from build123d import *

# Parameters (mm, degrees)
EXTRUDE_1_DEPTH     = 15
EXTRUDE_1_2_DEPTH   = 15
EXTRUDE_2_DEPTH     = 4
EXTRUDE_5_DEPTH     = 4
SKETCH_8_W          = 5
SKETCH_8_H          = 5
EXTRUDE_6_DEPTH     = 37
SKETCH_9_W          = 4
SKETCH_9_H          = 5
EXTRUDE_7_DEPTH     = 60
EXTRUDE_8_DEPTH     = 5
FILLET_1_R          = 1
FILLET_2_R          = 1
SKETCH_11_W         = 94.407997399
SKETCH_11_H         = 0.2
CUT_EXTRUDE_1_DEPTH = 61


with BuildPart() as part:
    # Sketch 1 → Extrude 1 (new body)
    with BuildSketch(Plane.XY):
        with BuildLine():
            Line((539.301234579, 452.744075086), (539.301234579, 447.744075086))
            Line((539.301234579, 447.744075086), (534.301234579, 447.744075086))
            ThreePointArc((534.301234579, 447.744075086), (531.801234579, 450.244075086), (534.301234579, 452.744075086))
            Line((534.301234579, 452.744075086), (539.301234579, 452.744075086))
        make_face()
    extrude(amount=-EXTRUDE_1_DEPTH)



with BuildPart() as body_2:
    # Sketch 1 → Extrude 1 2 (new body)
    with BuildSketch(Plane.XY):
        with BuildLine():
            Line((459.301234579, 452.744075086), (459.301234579, 447.744075086))
            Line((459.301234579, 447.744075086), (454.301234579, 447.744075086))
            ThreePointArc((454.301234579, 447.744075086), (451.801234579, 450.244075086), (454.301234579, 452.744075086))
            Line((454.301234579, 452.744075086), (459.301234579, 452.744075086))
        make_face()
    extrude(amount=-EXTRUDE_1_2_DEPTH)


with BuildPart() as part_1:
    add(part.part)

    add(body_2.part)  # Extrude 2 merges body 2
    # Sketch 2 → Extrude 2 (add)
    with BuildSketch(Plane(origin=(0, 0, -15), x_dir=(-1, 0, 0), z_dir=(0, 0, -1))):
        with BuildLine():
            Line((-529.301234579, 452.744075086), (-534.301234579, 452.744075086))
            Line((-534.301234579, 452.744075086), (-539.301234579, 452.744075086))
            Line((-539.301234579, 452.744075086), (-539.301234579, 447.744075086))
            Line((-539.301234579, 447.744075086), (-534.301234579, 447.744075086))
            Line((-534.301234579, 447.744075086), (-529.301234579, 447.744075086))
            ThreePointArc((-529.301234579, 447.744075086), (-526.801234579, 450.244075086), (-529.301234579, 452.744075086))
        make_face()
        with BuildLine():
            Line((-449.301234579, 452.744075086), (-459.301234579, 452.744075086))
            Line((-459.301234579, 452.744075086), (-459.301234579, 447.744075086))
            Line((-459.301234579, 447.744075086), (-449.301234579, 447.744075086))
            ThreePointArc((-449.301234579, 447.744075086), (-446.801234579, 450.244075086), (-449.301234579, 452.744075086))
        make_face()
    extrude(amount=EXTRUDE_2_DEPTH)

    # Sketch 7 → Extrude 5 (add)
    with BuildSketch(Plane.XY):
        with BuildLine():
            Line((539.301234579, 447.744075086), (454.301234579, 447.744075086))
            ThreePointArc((454.301234579, 447.744075086), (451.801234579, 450.244075086), (454.301234579, 452.744075086))
            Line((454.301234579, 452.744075086), (539.301234579, 452.744075086))
            Line((539.301234579, 452.744075086), (539.301234579, 447.744075086))
        make_face()
    extrude(amount=EXTRUDE_5_DEPTH)

    # Sketch 8 → Extrude 6 (add)
    with BuildSketch(Plane.XY.offset(4)):
        with Locations((536.801234579, 450.244075086)):
            Rectangle(SKETCH_8_W, SKETCH_8_H)
        with Locations((476.801234579, 450.244075086)):
            Rectangle(SKETCH_8_W, SKETCH_8_H)
    extrude(amount=EXTRUDE_6_DEPTH)

    # Sketch 9 → Extrude 7 (add)
    with BuildSketch(Plane.ZY.offset(-534.301234579)):
        with Locations((39, 450.244075086)):
            Rectangle(SKETCH_9_W, SKETCH_9_H)
    extrude(amount=EXTRUDE_7_DEPTH)

    # Sketch 10 → Extrude 8 (add)
    with BuildSketch(Plane.XZ.offset(-447.744075086)):
        Polygon((474.301234579, 4), (469.301234579, 4), (474.301234579, 9), align=None)
    extrude(amount=-EXTRUDE_8_DEPTH)

    # Fillet 1
    fillet_1_edges = [part_1.edges().sort_by_distance(p)[0] for p in [
        (534.301234579, 450.244075086, 4),
        (479.301234579, 450.244075086, 4),
        (479.301234579, 450.244075086, 37),
        (534.301234579, 450.244075086, 37),
    ]]
    fillet(fillet_1_edges, radius=FILLET_1_R)

    # Fillet 2
    fillet_2_edges = [part_1.edges().sort_by_distance(p)[0] for p in [
        (469.301234579, 450.244075086, 4),
        (474.301234579, 450.244075086, 9),
        (539.301234579, 450.244075086, 41),
        (474.301234579, 450.244075086, 41),
    ]]
    fillet(fillet_2_edges, radius=FILLET_2_R)

    # Sketch 11 → Cut-Extrude 1 (cut, through all)
    with BuildSketch(Plane.XY.offset(41)):
        with Locations((493.383672974, 452.644075086)):
            Rectangle(SKETCH_11_W, SKETCH_11_H)
        with Locations((493.383672974, 447.844075086)):
            Rectangle(SKETCH_11_W, SKETCH_11_H)
    extrude(amount=-CUT_EXTRUDE_1_DEPTH, mode=Mode.SUBTRACT)


solid = part_1.part
Here's how the part is built. I have some questions about the finished solid (model axes, mm). A direction names the side the tool comes from. Round coordinates to 2 decimals unless told otherwise and drop trailing zeros. Write each loop counter-clockwise with the first axis right and the second up, starting at its lowest first coordinate (ties: lowest second). Pieces come first, ordered by that corner, then holes.
1. I need wall thicknesses on L1, parallel to Z at x = 517, y = 452.2; L2, parallel to X at y = 451.9, z = 28.5; L3, parallel to Z at x = 457.5, y = 448.9. Which ranges of each line are inside material? Lowest first, please.
2. Will this pin go through, and if not, where does the flat tip stop? pin 1 Ø2.5 at (y, z) = (449.5, 17.5) entering from -X.
3. Suppose I cut it at B-B (z = -9). List the corners of the cut face in (x, y) for me, and give its area (3 significant figures).
4. Suppose I cut it at C-C (y = 449.4). List the corners of the cut face in (x, z) for me.
5. Suppose I cut it at D-D (x = 456). List the corners of the cut face in (y, z) for me, and give its area (3 significant figures).
6. For faces 4 (the flat face through (459.301, 450, -9)), 5 (the flat face through (507, 450, 37)), 6 (the cylindrical face through (451.8, 450.2, -5.6)), 7 (the flat face through (474.301, 450, 24)), 8 (the cylindrical face through (526.8, 450.2, -17)), which set-ups out of +Z, -Z, +X, -X, +Y, -Y let a thin tool reach every point of the face, with its end or its side?
7. Suppose I cut it at A-A (x = 490). List the corners of the cut face in (y, z) for me.
8. If we mould it in two halves opening along Z, with no side actions, what happens to faces 1 (the flat face through (504, 447.944, 2)), 2 (the flat face through (453, 450, -19)), 3 (the flat face through (529, 450, -15))? For each: released by +Z, released by -Z, zero draft, split by the parting line, or undercut.
Answer sheet:
1. L1: z = 0 to 4, 37 to 41
1. L2: x = 474.3 to 479.3, 534.3 to 539.3
1. L3: z = -19 to 4
2. pin 1: stops at x = 474.3
3. outline: (453.32, 447.94) - (459.3, 447.94) - (459.3, 452.54) - (453.32, 452.54) arc R2.5 ccw to start; (533.32, 447.94) - (539.3, 447.94) - (539.3, 452.54) - (533.32, 452.54) arc R2.5 ccw to start
3. area: 65.1 mm2
4. outline: (446.95, -19) - (459.3, -19) - (459.3, 0) - (531.95, 0) - (531.95, -15) - (526.95, -15) - (526.95, -19) - (539.3, -19) - (539.3, 40) arc R1 ccw to (538.3, 41) - (475.3, 41) arc R1 ccw to (474.3, 40) - (474.3, 9.41) arc R1 cw to (474.01, 8.71) - (469.59, 4.29) arc R1 cw to (468.89, 4) - (451.95, 4) - (451.95, -15) - (446.95, -15) - close; hole (479.3, 5) arc R1 ccw to (480.3, 4) - (533.3, 4) arc R1 ccw to (534.3, 5) - (534.3, 36) arc R1 ccw to (533.3, 37) - (480.3, 37) arc R1 ccw to (479.3, 36) - close
5. outline: (447.94, -19) - (452.54, -19) - (452.54, 4) - (447.94, 4) - close
5. area: 106 mm2
6. face 4: -Z, +Y, -Y
6. face 5: +Y, -Y
6. face 6: +Z, -X
6. face 7: +Z, -X, +Y, -Y
6. face 8: -Z
7. outline: (447.94, 0) - (452.54, 0) - (452.54, 4) - (447.94, 4) - close; (447.94, 37) - (452.54, 37) - (452.54, 41) - (447.94, 41) - close
8. face 1: zero draft
8. face 2: released by -Z
8. face 3: undercut
